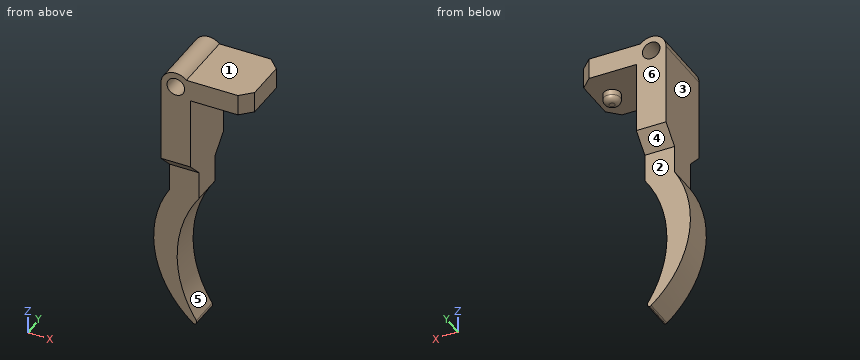
```python
from build123d import *

# Parameters (mm, degrees)
F0_R        = 1.6
F1_DEPTH    = 5.8
F0_W        = 5.4
F0_H        = 5
F2_DEPTH    = 2.8
F3_SIZE     = 2.99999
F4_R        = 1.5
F5_DEPTH    = 2
F6_R        = 1
F7_T1_DEPTH = 6.481505829
F7_T3_DEPTH = 10.3311661503
F8_SIZE     = 2


# Not quite as in the source:
# - a fillet or chamfer that OpenCascade refuses, or shapes differently, is made with other operations: its cross-section is extruded or revolved along the edge and cut away or added
# - a fillet or chamfer is up to 0.001 mm smaller than in the source, because OpenCascade refuses the exact size


with BuildPart() as f1:
    # F0 (on Front) → F1 (new body, symmetric)
    with BuildSketch(Plane.XZ):
        with BuildLine():
            ThreePointArc((1.9183326093, -1.9), (2.4969479415, -1.0272540958), (2.7, 0))
            ThreePointArc((2.7, 0), (2.4969479415, 1.0272540958), (1.9183326093, 1.9))
            ThreePointArc((1.9183326093, 1.9), (-1.0272540958, 2.4969479415), (-2.7, 0))
            ThreePointArc((-2.7, 0), (-1.0272540958, -2.4969479415), (1.9183326093, -1.9))
        make_face()
        Circle(F0_R, mode=Mode.SUBTRACT)
        with BuildLine():
            ThreePointArc((1.9183326093, 1.9), (2.4969479415, 1.0272540958), (2.7, 0))
            ThreePointArc((2.7, 0), (2.4969479415, -1.0272540958), (1.9183326093, -1.9))
            Line((1.9183326093, -1.9), (2.7, -1.9))
            Line((2.7, -1.9), (13.3, -1.9))
            Line((13.3, -1.9), (13.3, 1.9))
            Line((13.3, 1.9), (1.9183326093, 1.9))
        make_face()
        with BuildLine():
            Line((2.7, -1.9), (1.9183326093, -1.9))
            ThreePointArc((1.9183326093, -1.9), (-1.0272540958, -2.4969479415), (-2.7, 0))
            Line((-2.7, 0), (-2.7, -17.9))
            Line((-2.7, -17.9), (2.7, -17.9))
            Line((2.7, -17.9), (2.7, -1.9))
        make_face()
    extrude(amount=F1_DEPTH, both=True)

    # F0 (on Front) → F2 (join, symmetric)
    with BuildSketch(Plane.XZ):
        with BuildLine():
            Line((2.7, -22.9), (-2.7, -22.9))
            ThreePointArc((-2.7, -22.9), (-5.2874639524, -36.2425936556), (1.7, -47.9))
            Line((1.7, -47.9), (2.7, -47.9))
            ThreePointArc((2.7, -47.9), (-1.3071443155, -35.4), (2.7, -22.9))
        make_face()
        with Locations((0, -20.4)):
            Rectangle(F0_W, F0_H)
    extrude(amount=F2_DEPTH, both=True)

    # F3 (size 3 in the source; OpenCascade refuses exactly that, so slightly less here)
    f3_edges = [f1.edges().sort_by_distance(p)[0] for p in [
        (0, -5.8, -17.9),
        (0, 5.8, -17.9),
    ]]
    chamfer(f3_edges, length=F3_SIZE)

    # F4 (on face) → F5 (join)
    with BuildSketch(Plane(origin=(0, 0, -1.9), x_dir=(1, 0, 0), z_dir=(0, 0, -1))):
        with Locations((10.1, 0)):
            Circle(F4_R)
    extrude(amount=F5_DEPTH)

    # F6
    f6_edges = [f1.edges().sort_by_distance(p)[0] for p in [
        (8.6, 0, -3.9),
    ]]
    fillet(f6_edges, radius=F6_R)

    # F7: fillet of radius 0.5 on 2 edges, made by hand

    # F7_s2 → F7_t1 (cut)
    with BuildSketch(Plane.XZ.offset(-3.2407529145)):
        with BuildLine():
            ThreePointArc((1.8739659479, -47.9), (1.7085587408, -47.871847916), (1.561777764, -47.7905618233))
            ThreePointArc((1.561777764, -47.7905618233), (1.6307619466, -47.8454412332), (1.7, -47.9))
            Line((1.7, -47.9), (1.8739659479, -47.9))
        make_face()
    extrude(amount=F7_T1_DEPTH, mode=Mode.SUBTRACT)

    # F7_s4 → F7_t3 (cut)
    with BuildSketch(Plane.XZ.offset(-5.1655830752)):
        with BuildLine():
            ThreePointArc((2.1728369726, -47.1272727273), (2.1932913064, -47.6383656473), (1.7537667699, -47.9))
            Line((1.7537667699, -47.9), (2.7, -47.9))
            ThreePointArc((2.7, -47.9), (2.4322155262, -47.5165036692), (2.1728369726, -47.1272727273))
        make_face()
    extrude(amount=F7_T3_DEPTH, mode=Mode.SUBTRACT)

    # F8
    f8_edges = [f1.edges().sort_by_distance(p)[0] for p in [
        (13.3, -5.8, 0),
        (13.3, 5.8, 0),
    ]]
    chamfer(f8_edges, length=F8_SIZE)


solid = f1.part
```
Source: CAD feature listing. Evaluate the final solid. Frame: model axes, mm. Face numbers are marked on the shaded views. A direction names the side the tool comes from. Round coordinates to 2 decimals unless told otherwise and drop trailing zeros. Write each loop counter-clockwise with the first axis right and the second up, starting at its lowest first coordinate (ties: lowest second). Pieces come first, ordered by that corner, then holes. Notation, with made-up numbers: M 65,54 L 94,54 A24 cw 94,67 Z; hole C -19.75,57.5 d11. An arc over 180 degrees is marked long. Use CSV: the item, a comma, the result in double quotes. Start each with the question number.
Q1. Cut plane B-B on y = 2.25. Output: boundary loops of the cut face in (x, z).
Q2. First-contact query: P1, Ø6, axis at y = -0.5, z = -15, coming from the -X side; P2, Ø6, axis at x = 6.5, y = 0.5, coming from the +Z side; P3, Ø0.5, axis at x = 10, y = 0, coming from the -Z side. Flat tips, straight axial feed; report the tip coordinate or a pass-through.
Q3. Pull-direction query (Z, two-part tool) for the marked faces 4, 5 and 6; classes: +Z half, -Z half, draft (parallel to the pull), parting line (faces both ways), or undercut.
Q4. Cut plane C-C on z = -8. Output: boundary loops of the cut face in (x, y), plus the area to 3 significant figures.
Q5. Line query: line 1 (Z direction, x = 4.5, y = 0.75); line 2 (Y direction, x = -3.5, z = -35); line 3 (X direction, y = 2.75, z = -16). Output: solid intervals per line, ascending. Write a range as from..to.
Q6. Access query for the marked faces 1, 2 and 3. Directions: +Z, -Z, +X, -X, +Y, -Y. A direction counts if a zero-diameter tool reaches every point of the face in a straight line with its end or side. Return the directions, or none.
Q7. Cut plane A-A on x = 0. Count the separate pieces of the cut face and the enclosed holes in it, plus the area to 3 significant figures.
Q8. Cut plane D-D on x = -3.25. Output: boundary loops of the cut face in (y, z).
Results found:
1,outline,"M -2.7,-22.9 A19 ccw 1.56,-47.79 A0.5 ccw 1.81,-47.9 A0.5 ccw 2.17,-47.13 A21.5 cw 2.7,-22.9 L 2.7,-1.9 L 13.3,-1.9 L 13.3,1.9 L 1.92,1.9 A2.7 ccw -2.7,0 Z; hole C 0,0 d3.2"
2,P1,"x = -2.7"
2,P2,"z = 1.9"
2,P3,"z = -3.9"
3,face 4,"-Z half"
3,face 5,"undercut"
3,face 6,"draft"
4,outline,"M -2.7,-5.8 L 2.7,-5.8 L 2.7,5.8 L -2.7,5.8 Z"
4,area,"62.6 mm^2"
5,line 1,"-1.9..1.9"
5,line 2,"-2.8..2.8"
5,line 3,"-2.7..2.7"
6,face 1,"+Z, +X, +Y, -Y"
6,face 2,"-Z, +X, -X, +Y"
6,face 3,"+Z, -X, +Y, -Y"
7,separate pieces,"3"
7,enclosed holes,"0"
7,area,"270 mm^2"
8,outline,"M -2.8,-42.06 L 2.8,-42.06 L 2.8,-23.84 L -2.8,-23.84 Z"
